Can you work these out from the model? Positions are in its coordinate system, mm. A direction names the side the tool comes from. Coordinates: 2 decimals unless noted, no trailing zeros. Order: outer loops, then holes, each group sorted by start corner. A loop starts at its lowest first (then second) coordinate and runs counter-clockwise, first axis right, second up. Notation, with made-up numbers: (59.5, 3) - (108.5, 3) arc R22 ccw to (108.5, 16) - close; hole circle Ø1 at (-11, 36). An arc over 180 degrees is marked (long way). Return JSON: item names as keys, results as strings. Group by question number.
1) Imagine slicing it at B-B (y = -5.5). Write out the boundary of the cut face in (x, z) (1 decimal), and give its area (3 significant figures).
2) If I drill on line 1 along Z through (x, y) = (0, -10.5); line 2 along X through (y, z) = (1.5, 0); line 3 along Y through (x, z) = (3, 10.5), over which ranges is the centre line in solid material (lowest first)?
3) If we mould it in two halves opening along X, with no side actions, what happens to faces 3 (the face through (-13.178, 0.276, -0.032)), 4 (the face through (6.561, 0.276, 11.428)), 5 (the face through (-0.34, -4.95, -1.55))? For each: pulls with the +X half, pulls with the -X half, needs draft (parallel to the pull), parting line crosses it, or undercut.
4) For pin 1 Ø10 at (x, y) = (10, -9) entering from -Z; pin 2 Ø3 at (x, y) = (10, 6) entering from -Z; pin 3 Ø6 at (x, z) = (-11, -4.5) entering from -Y, each with a flat end and sliding along its axis, tell me the tip position at first contact or that it passes through.
5) Imagine slicing it at A-A (y = 7.5). Write out the boundary of the cut face in (x, z) (1 decimal), and give its area (3 significant figures).
6) Which directions (+Z, -Z, +X, -X, +Y, -Y) give clear straight access to the entire face, cutting with the end or side of a thin tool? Please do faces 1 (the face through (3, -15, -6)), 2 (the face through (0, 5, 12.7)).
```python
from build123d import *

# Parameters (mm, degrees)
SALIENTE_EXTRUIR3_DEPTH = 10
CROQUIS5_OUTSIDE_W      = 73.984
CROQUIS5_OUTSIDE_H      = 70.054
CROQUIS5_OUTSIDE_R      = 12.7
CORTAR_EXTRUIR4_DEPTH   = 10
CORTAR_EXTRUIR4_TAPER   = 60
CROQUIS6_OUTSIDE_W      = 73.984
CROQUIS6_OUTSIDE_H      = 70.054
CROQUIS6_OUTSIDE_R      = 12.7
CORTAR_EXTRUIR5_DEPTH   = 10
CORTAR_EXTRUIR5_TAPER   = 60
CROQUIS7_R              = 9
SALIENTE_EXTRUIR4_DEPTH = 15
CHAFL_N1_SIZE           = 2
CROQUIS8_R              = 1.5875
CORTAR_EXTRUIR6_DEPTH   = 26
CHAFL_N2_SIZE           = 0.5
CROQUIS9_R              = 6.35
SALIENTE_EXTRUIR5_DEPTH = 4
CHAFL_N4_SIZE           = 1
CROQUIS10_R             = 1.5875
CORTAR_EXTRUIR7_DEPTH   = 14


with BuildPart() as part:
    # Croquis1 → Saliente-Extruir3 (new body)
    with BuildSketch(Plane(origin=(0, 0, 0), x_dir=(1, 0, 0), z_dir=(0, 1, 0))):
        Polygon((14.664696837, 0), (7.332348419, 12.7), (-7.332348419, 12.7), (-14.664696837, 0), (-7.332348419, -12.7), (7.332348419, -12.7), align=None)
    extrude(amount=SALIENTE_EXTRUIR3_DEPTH)

    # Croquis5 outside → Cortar-Extruir4 (cut)
    with BuildSketch(Plane.XZ):
        Rectangle(CROQUIS5_OUTSIDE_W, CROQUIS5_OUTSIDE_H)
        Circle(CROQUIS5_OUTSIDE_R, mode=Mode.SUBTRACT)
    extrude(amount=-CORTAR_EXTRUIR4_DEPTH, taper=CORTAR_EXTRUIR4_TAPER, mode=Mode.SUBTRACT)

    # Croquis6 outside → Cortar-Extruir5 (cut)
    with BuildSketch(Plane(origin=(0, 10, 0), x_dir=(1, 0, 0), z_dir=(0, 1, 0))):
        Rectangle(CROQUIS6_OUTSIDE_W, CROQUIS6_OUTSIDE_H)
        Circle(CROQUIS6_OUTSIDE_R, mode=Mode.SUBTRACT)
    extrude(amount=-CORTAR_EXTRUIR5_DEPTH, taper=CORTAR_EXTRUIR5_TAPER, mode=Mode.SUBTRACT)

    # Croquis7 → Saliente-Extruir4 (add)
    with BuildSketch(Plane.XZ):
        Circle(CROQUIS7_R)
    extrude(amount=SALIENTE_EXTRUIR4_DEPTH)

    # Chaflán1
    chafl_n1_edges = [part.edges().sort_by_distance(p)[0] for p in [
        (-9, -15, 0),
    ]]
    chamfer(chafl_n1_edges, length=CHAFL_N1_SIZE)

    # Croquis8 → Cortar-Extruir6 (cut)
    with BuildSketch(Plane(origin=(0, 10, 0), x_dir=(1, 0, 0), z_dir=(0, 1, 0))):
        Circle(CROQUIS8_R)
    extrude(amount=-CORTAR_EXTRUIR6_DEPTH, mode=Mode.SUBTRACT)

    # Chaflán2
    chafl_n2_edges = [part.edges().sort_by_distance(p)[0] for p in [
        (-1.5875, 10, 0),
    ]]
    chamfer(chafl_n2_edges, length=CHAFL_N2_SIZE)

    # Croquis9 → Saliente-Extruir5 (add)
    with BuildSketch(Plane.XZ.offset(15)):
        Circle(CROQUIS9_R)
    extrude(amount=SALIENTE_EXTRUIR5_DEPTH)

    # Chaflán4
    chafl_n4_edges = [part.edges().sort_by_distance(p)[0] for p in [
        (-6.35, -19, 0),
    ]]
    chamfer(chafl_n4_edges, length=CHAFL_N4_SIZE)

    # Croquis10 → Cortar-Extruir7 (cut)
    with BuildSketch(Plane.XZ.offset(19)):
        Circle(CROQUIS10_R)
    extrude(amount=-CORTAR_EXTRUIR7_DEPTH, mode=Mode.SUBTRACT)


solid = part.part
```
Calculated:
{
 "1": {"outline": "circle Ø18 at (0, 0); hole circle Ø3.2 at (0, 0)", "area": "247 mm2"},
 "2": {"line 1": "-9 to -1.59, 1.59 to 9", "line 2": "-14.66 to -1.59, 1.59 to 14.66", "line 3": "0 to 10"},
 "3": {"face 3": "pulls with the -X half", "face 4": "pulls with the +X half", "face 5": "undercut"},
 "4": {"pin 1": "z = -7.48", "pin 2": "z = -10.68", "pin 3": "y = -13.12"},
 "5": {"outline": "(-14.7, 0) - (-7.3, -12.7) - (7.3, -12.7) - (14.7, 0) - (7.3, 12.7) - (-7.3, 12.7) - close; hole circle Ø3.2 at (0, 0)", "area": "551 mm2"},
 "6": {"face 1": "-Y", "face 2": "+Z, +X, -X, +Y, -Y"}
}
